Design review of the part built by this model. Coordinates are the model's own, in mm. A direction names the side the tool comes from. Give positions to 0.01 mm unless a question says otherwise; leave off trailing zeros. Write each loop counter-clockwise with the first axis right and the second up, starting at its lowest first coordinate (ties: lowest second). Pieces come first, ordered by that corner, then holes. Notation, with made-up numbers: (50, -2) -> (93, -2) arc R27 cw to (93, 25) -> close; hole circle Ø8 at (79.25, 67). An arc over 180 degrees is marked (long way). Write each question's results on one line, items separated by ' | '. Start each with the question number.
(1) Take a section at A-A (z = 18.5). State the section outline as (x, y) points.
(2) Mouldability with a two-part tool opening along Z and no side actions: class faces 3 (the face through (0, 0, 0)), 4 (the face through (-0.14, 1.09, 32.85)), 5 (the face through (-0.27, -1.22, 16.83)), 6 (the face through (0, 0, 34)) as released by +Z, released by -Z, zero draft, split by the parting line, or undercut.
(3) To check wall thickness, follow probe 1 along Z at (x, y) = (-0.95, 0.7); probe 2 along Y at (x, z) = (0.1, 20); probe 3 along X at (y, z) = (-0.6, 2.5). State the ranges of each line that lie inside material, in increasing order.
(4) For faces 1 (the face through (1.05, 0.33, 1.2)), 2 (the face through (-0.27, -1.22, 0.54)), list the 3-axis set-ups (+Z, -Z, +X, -X, +Y, -Y) from which the entire face can be reached by the end or side of a thin tool; tool diameter is ignored.
from build123d import *

# Parameters (mm, degrees)
SKETCH_1_R          = 1.25
EXTRUDE_1_DEPTH     = 34
SKETCH_2_R          = 1.25
SKETCH_2_R_2        = 1.1
CUT_EXTRUDE_1_DEPTH = 0.4
SKETCH_3_R          = 1.25
SKETCH_3_R_2        = 1.1
CUT_EXTRUDE_2_DEPTH = 0.3
CHAMFER_1_SIZE      = 0.1


with BuildPart() as part:
    # 草图1 → 凸台-拉伸1 (new body)
    with BuildSketch(Plane.XY):
        Circle(SKETCH_1_R)
    extrude(amount=EXTRUDE_1_DEPTH)

    # 草图2 → 切除-拉伸1 (cut)
    with BuildSketch(Plane.XY.offset(1)):
        Circle(SKETCH_2_R)
        Circle(SKETCH_2_R_2, mode=Mode.SUBTRACT)
    extrude(amount=CUT_EXTRUDE_1_DEPTH, mode=Mode.SUBTRACT)

    # 草图3 → 切除-拉伸2 (cut)
    with BuildSketch(Plane.XY.offset(33)):
        Circle(SKETCH_3_R)
        Circle(SKETCH_3_R_2, mode=Mode.SUBTRACT)
    extrude(amount=-CUT_EXTRUDE_2_DEPTH, mode=Mode.SUBTRACT)

    # 倒角1
    chamfer_1_edges = [part.edges().sort_by_distance(p)[0] for p in [
        (-1.25, 0, 0),
        (-1.25, 0, 34),
    ]]
    chamfer(chamfer_1_edges, length=CHAMFER_1_SIZE)


solid = part.part
Report:
1) outline: circle Ø2.5 at (0, 0)
2) face 3: released by -Z | face 4: undercut | face 5: zero draft | face 6: released by +Z
3) probe 1: 0.03 to 1, 1.4 to 32.7, 33 to 33.97 | probe 2: -1.25 to 1.25 | probe 3: -1.1 to 1.1
4) face 1: none | face 2: +Z, -Z
